Design review of the part built by this model. Coordinates are the model's own, in mm. Round coordinates to 2 decimals unless told otherwise and drop trailing zeros. Write each loop counter-clockwise with the first axis right and the second up, starting at its lowest first coordinate (ties: lowest second). Pieces come first, ordered by that corner, then holes. Notation, with made-up numbers: (-21, 24) - (25, 24) arc R13 cw to (25, 42) - close; hole circle Ø2 at (64.5, -12). An arc over 180 degrees is marked (long way). Use one line per item in the form item = value.
```python
from build123d import *

# Parameters (mm, degrees)
F0_W     = 914.4
F0_H     = 609.6
F0_R     = 25.4
F1_DEPTH = 25.4


with BuildPart() as f1:
    # F0 (on Top) → F1 (new body)
    with BuildSketch(Plane.XY):
        with Locations((355.6, 178.164508)):
            Rectangle(F0_W, F0_H)
        with Locations((0, -25.035492)):
            Circle(F0_R, mode=Mode.SUBTRACT)
        with Locations((101.6, -25.035492)):
            Circle(F0_R, mode=Mode.SUBTRACT)
        with Locations((203.2, -25.035492)):
            Circle(F0_R, mode=Mode.SUBTRACT)
        with Locations((304.8, -25.035492)):
            Circle(F0_R, mode=Mode.SUBTRACT)
        with Locations((0, 76.564508)):
            Circle(F0_R, mode=Mode.SUBTRACT)
        with Locations((101.6, 76.564508)):
            Circle(F0_R, mode=Mode.SUBTRACT)
        with Locations((0, 178.164508)):
            Circle(F0_R, mode=Mode.SUBTRACT)
        with Locations((101.6, 178.164508)):
            Circle(F0_R, mode=Mode.SUBTRACT)
        with Locations((203.2, 76.564508)):
            Circle(F0_R, mode=Mode.SUBTRACT)
        with Locations((304.8, 76.564508)):
            Circle(F0_R, mode=Mode.SUBTRACT)
        with Locations((203.2, 178.164508)):
            Circle(F0_R, mode=Mode.SUBTRACT)
        with Locations((406.4, -25.035492)):
            Circle(F0_R, mode=Mode.SUBTRACT)
        with Locations((508, -25.035492)):
            Circle(F0_R, mode=Mode.SUBTRACT)
        with Locations((609.6, -25.035492)):
            Circle(F0_R, mode=Mode.SUBTRACT)
        with Locations((711.2, -25.035492)):
            Circle(F0_R, mode=Mode.SUBTRACT)
        with Locations((406.4, 76.564508)):
            Circle(F0_R, mode=Mode.SUBTRACT)
        with Locations((508, 76.564508)):
            Circle(F0_R, mode=Mode.SUBTRACT)
        with Locations((406.4, 178.164508)):
            Circle(F0_R, mode=Mode.SUBTRACT)
        with Locations((508, 178.164508)):
            Circle(F0_R, mode=Mode.SUBTRACT)
        with Locations((609.6, 76.564508)):
            Circle(F0_R, mode=Mode.SUBTRACT)
        with Locations((711.2, 76.564508)):
            Circle(F0_R, mode=Mode.SUBTRACT)
        with Locations((0, 279.764508)):
            Circle(F0_R, mode=Mode.SUBTRACT)
        with Locations((101.6, 279.764508)):
            Circle(F0_R, mode=Mode.SUBTRACT)
        with Locations((304.8, 178.164508)):
            Circle(F0_R, mode=Mode.SUBTRACT)
        with Locations((203.2, 279.764508)):
            Circle(F0_R, mode=Mode.SUBTRACT)
        with Locations((304.8, 279.764508)):
            Circle(F0_R, mode=Mode.SUBTRACT)
        with Locations((0, 381.364508)):
            Circle(F0_R, mode=Mode.SUBTRACT)
        with Locations((101.6, 381.364508)):
            Circle(F0_R, mode=Mode.SUBTRACT)
        with Locations((203.2, 381.364508)):
            Circle(F0_R, mode=Mode.SUBTRACT)
        with Locations((304.8, 381.364508)):
            Circle(F0_R, mode=Mode.SUBTRACT)
        with Locations((406.4, 279.764508)):
            Circle(F0_R, mode=Mode.SUBTRACT)
        with Locations((508, 279.764508)):
            Circle(F0_R, mode=Mode.SUBTRACT)
        with Locations((609.6, 178.164508)):
            Circle(F0_R, mode=Mode.SUBTRACT)
        with Locations((711.2, 178.164508)):
            Circle(F0_R, mode=Mode.SUBTRACT)
        with Locations((609.6, 279.764508)):
            Circle(F0_R, mode=Mode.SUBTRACT)
        with Locations((711.2, 279.764508)):
            Circle(F0_R, mode=Mode.SUBTRACT)
        with Locations((406.4, 381.364508)):
            Circle(F0_R, mode=Mode.SUBTRACT)
        with Locations((508, 381.364508)):
            Circle(F0_R, mode=Mode.SUBTRACT)
        with Locations((609.6, 381.364508)):
            Circle(F0_R, mode=Mode.SUBTRACT)
        with Locations((711.2, 381.364508)):
            Circle(F0_R, mode=Mode.SUBTRACT)
    extrude(amount=F1_DEPTH)


solid = f1.part
```
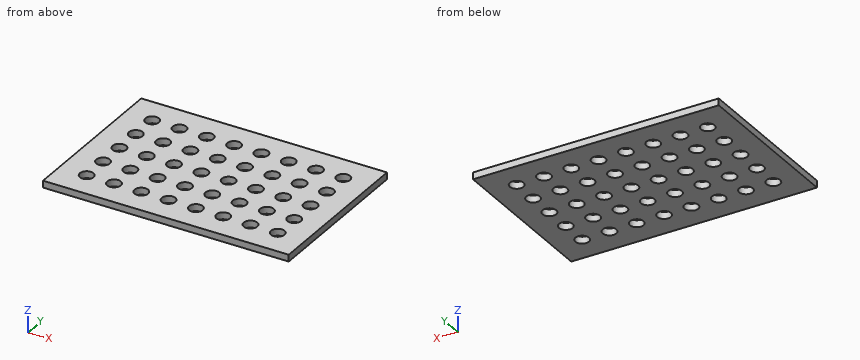
Q1. To check wall thickness, follow line 1 along Y through (x, z) = (203.2, 10.25); line 2 along Y through (x, z) = (17.5, 3.75) (1 decimal). State the ranges of each line that lie inside material, in increasing order. Write a range as from..to.
Calculated:
line_1 = -126.64..-50.44, 0.36..51.16, 101.96..152.76, 203.56..254.36, 305.16..355.96, 406.76..482.96
line_2 = -126.6..-43.4, -6.6..58.2, 95..159.8, 196.6..261.4, 298.2..363, 399.8..483
Q2. We need section A-A on x = 609.6. Write out the cut boundary in (y, z), then the cut area to 3 significant figures.
Calculated:
outline = (-126.64, 0) - (-50.44, 0) - (-50.44, 25.4) - (-126.64, 25.4) - close; (0.36, 0) - (51.16, 0) - (51.16, 25.4) - (0.36, 25.4) - close; (101.96, 0) - (152.76, 0) - (152.76, 25.4) - (101.96, 25.4) - close; (203.56, 0) - (254.36, 0) - (254.36, 25.4) - (203.56, 25.4) - close; (305.16, 0) - (355.96, 0) - (355.96, 25.4) - (305.16, 25.4) - close; (406.76, 0) - (482.96, 0) - (482.96, 25.4) - (406.76, 25.4) - close
area = 9,030 mm2
Q3. We need section B-B on x = 106. Write out the cut boundary in (y, z).
Calculated:
outline = (-126.64, 0) - (-50.05, 0) - (-50.05, 25.4) - (-126.64, 25.4) - close; (-0.02, 0) - (51.55, 0) - (51.55, 25.4) - (-0.02, 25.4) - close; (101.58, 0) - (153.15, 0) - (153.15, 25.4) - (101.58, 25.4) - close; (203.18, 0) - (254.75, 0) - (254.75, 25.4) - (203.18, 25.4) - close; (304.78, 0) - (356.35, 0) - (356.35, 25.4) - (304.78, 25.4) - close; (406.38, 0) - (482.96, 0) - (482.96, 25.4) - (406.38, 25.4) - close
Q4. We need section C-C on z = 13.5. State how many separate pieces and enclosed holes the cut face has, then the cut area to 3 significant figures.
Calculated:
separate_pieces = 1
enclosed_holes = 40
area = 476,000 mm2
